```python
from build123d import *

# Parameters (mm, degrees)
SKETCH_1_R          = 2
EXTRUDE_1_DEPTH     = 13
SKETCH_2_W          = 7
SKETCH_2_H          = 34.84138361
CUT_EXTRUDE_1_DEPTH = 193.919672403
SKETCH_3_W          = 10.3
SKETCH_3_H          = 7.1
CUT_EXTRUDE_2_DEPTH = 60


with BuildPart() as part:
    # 草图1 → 凸台-拉伸1 (new body)
    with BuildSketch(Plane.XY):
        with BuildLine():
            Line((54, -72), (75, -72))
            ThreePointArc((75, -72), (78.535533906, -73.464466094), (80, -77))
            Line((80, -77), (80, -107))
            Line((80, -107), (-80, -107))
            Line((-80, -107), (-80, -77))
            ThreePointArc((-80, -77), (-78.535533906, -73.464466094), (-75, -72))
            Line((-75, -72), (-54, -72))
            ThreePointArc((-54, -72), (0, -90), (54, -72))
        make_face()
        with Locations(Location((-64.83247643, -87, 0), (0, 0, 180))):
            Circle(SKETCH_1_R, mode=Mode.SUBTRACT)
        with Locations(Location((64.83247643, -87, 0), (0, 0, 180))):
            Circle(SKETCH_1_R, mode=Mode.SUBTRACT)
    extrude(amount=EXTRUDE_1_DEPTH)

    # 草图2 → 切除-拉伸1 (cut, through all)
    with BuildSketch(Plane(origin=(80, 0, 0), x_dir=(0, 0, -1), z_dir=(1, 0, 0))):
        with Locations((-6.5, -87.579308195)):
            Rectangle(SKETCH_2_W, SKETCH_2_H)
    extrude(amount=-CUT_EXTRUDE_1_DEPTH, mode=Mode.SUBTRACT)

    # 草图3 → 切除-拉伸2 (cut)
    with BuildSketch(Plane.XY.offset(13)):
        with Locations((-64.83247643, -103.45)):
            Rectangle(SKETCH_3_W, SKETCH_3_H)
        with Locations((64.83247643, -103.45)):
            Rectangle(SKETCH_3_W, SKETCH_3_H)
    extrude(amount=-CUT_EXTRUDE_2_DEPTH, mode=Mode.SUBTRACT)


solid = part.part
```
Input: part model. Units: mm. Frame: model coordinates. A direction names the side the tool comes from. Round coordinates to 2 decimals unless told otherwise and drop trailing zeros. Loops run counter-clockwise (first coordinate to the right, second up) from the corner with the lowest first, then second, coordinate; pieces in that order, holes last. Notation, with made-up numbers: (-22.75, 61.5) -> (2.25, 61.5) arc R13 ccw to (2.25, 75.5) -> close; hole circle Ø10 at (31, 33). An arc over 180 degrees is marked (long way). One line per item, written item: value.
(1) Set-up query: faces 4 (the face through (-0.811, -89.996, 11.479)), 5 (the face through (1, -92, 10)), 6 (the face through (65, -99.9, 2)). Return all of +Z, -Z, +X, -X, +Y, -Y with unobstructed straight access to the full face (end or side cutting, diameter ignored); none if empty.
Geometry check:
face 4: +Z, -Z, +Y
face 5: +X, -X, +Y
face 6: +Z, -Z, -Y
(2) Material intervals for line 1 (Z direction, x = 39, y = -96); line 2 (Y direction, x = -73, z = 3.75); line 3 (X direction, y = -77, z = 10.25), sorted ascending. Write a range as [from, to].
Geometry check:
line 1: [0, 3], [10, 13]
line 2: [-107, -105]
line 3: [-80, -46.59], [46.59, 80]
(3) Pin query (flat end, axial travel): pin 1 (2.5 mm diameter, centred on x = -66.5, z = 2, fed in from -Y); pin 2 (3.5 mm diameter, centred on x = -64.83, y = -87, fed in from -Z); pin 3 (5.5 mm diameter, centred on x = 11, z = 6, fed in from +Y). Return the tip coordinate at first contact, or that it passes through.
Geometry check:
pin 1: y = -99.9
pin 2: through
pin 3: y = -105
(4) Section C-C (y = -95.5). Return the cut outline in (x, z).
Geometry check:
outline: (-80, 0) -> (80, 0) -> (80, 3) -> (-80, 3) -> close; (-80, 10) -> (80, 10) -> (80, 13) -> (-80, 13) -> close
(5) Section A-A (y = -101.5). Return the cut outline in (x, z), plus the area to 3 significant figures.
Geometry check:
outline: (-80, 0) -> (-69.98, 0) -> (-69.98, 3) -> (-80, 3) -> close; (-80, 10) -> (-69.98, 10) -> (-69.98, 13) -> (-80, 13) -> close; (-59.68, 0) -> (59.68, 0) -> (59.68, 3) -> (-59.68, 3) -> close; (-59.68, 10) -> (59.68, 10) -> (59.68, 13) -> (-59.68, 13) -> close; (69.98, 0) -> (80, 0) -> (80, 3) -> (69.98, 3) -> close; (69.98, 10) -> (80, 10) -> (80, 13) -> (69.98, 13) -> close
area: 836 mm2
(6) Section B-B (z = 5). Return the cut outline in (x, y), plus the area to 3 significant figures.
Geometry check:
outline: (-80, -107) -> (-69.98, -107) -> (-69.98, -105) -> (-80, -105) -> close; (-59.68, -107) -> (59.68, -107) -> (59.68, -105) -> (-59.68, -105) -> close; (69.98, -107) -> (80, -107) -> (80, -105) -> (69.98, -105) -> close
area: 279 mm2
(7) Mould query, pull axis X, two halves, no side actions, for faces 1 (the face through (65.093, -88.983, 11.479)), 2 (the face through (64, -72, 1)), 3 (the face through (-80, -92, 11)). Classes: pulls with the +X half, pulls with the -X half, needs draft (parallel to the pull), parting line crosses it, or undercut.
Geometry check:
face 1: undercut
face 2: needs draft
face 3: pulls with the -X half
(8) Section D-D (x = -51). Return the cut outline in (y, z), plus the area to 3 significant figures.
Geometry check:
outline: (-107, 0) -> (-74.16, 0) -> (-74.16, 3) -> (-105, 3) -> (-105, 10) -> (-74.16, 10) -> (-74.16, 13) -> (-107, 13) -> close
area: 211 mm2
